Design review of the part shown in the three views and the two pictorial views. Dimensions are in mm from the part's minimum x, y and z. A direction names the side the tool comes from. Round coordinates to 2 decimals unless told otherwise and drop trailing zeros. Write each loop counter-clockwise with the first axis right and the second up, starting at its lowest first coordinate (ties: lowest second). Pieces come first, ordered by that corner, then holes. Notation, with made-up numbers: (-40, -33.75) - (-16, -33.75) arc R22 ccw to (-16, -11.75) - close; hole circle Ø5 at (50.5, 78.5). An arc over 180 degrees is marked (long way). Use one line per item in the form item = value.
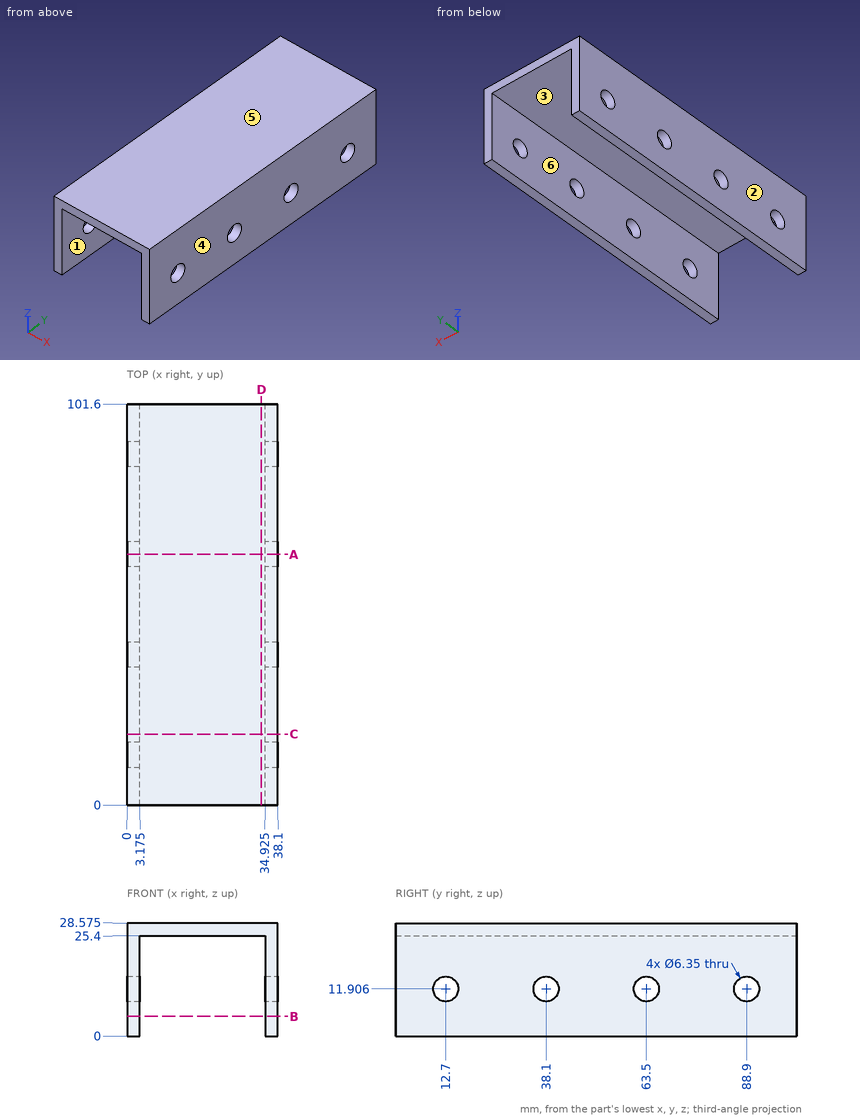
Q1. Draft analysis for pull direction X (two halves, no side actions). For the marked faces 3, 4, 5 and 6, state which applies: released by +X, released by -X, zero draft, split by the parting line, or undercut.
Calculated:
face_3 = undercut
face_4 = released by +X
face_5 = zero draft
face_6 = undercut
Q2. For P1, Ø4, axis at y = 63.5, z = 11.91, coming from the +X side; P2, Ø9.5, axis at x = 22.5, y = 33, coming from the -Z side, all flat-tipped, find the tip position at first contact; note any pin that passes through.
Calculated:
P1 = through
P2 = 25.4
Q3. We need section A-A on y = 63.5. Write out the cut boundary in (x, z) (1 decimal), then the cut area to 3 significant figures.
Calculated:
outline = (0, 0) - (3.2, 0) - (3.2, 8.7) - (0, 8.7) - close; (0, 15.1) - (3.2, 15.1) - (3.2, 25.4) - (34.9, 25.4) - (34.9, 15.1) - (38.1, 15.1) - (38.1, 28.6) - (0, 28.6) - close; (34.9, 0) - (38.1, 0) - (38.1, 8.7) - (34.9, 8.7) - close
area = 242 mm2
Q4. To check wall thickness, follow line 1 along X through (y, z) = (17.5, 5.5) (1 decimal); line 2 along Z through (x, y) = (16, 67.5) (1 decimal); line 3 along Y through (x, z) = (2, 13.5) (1 decimal). State the ranges of each line that lie inside material, in increasing order. Write a range as from..to.
Calculated:
line_1 = 0..3.2, 34.9..38.1
line_2 = 25.4..28.6
line_3 = 0..10, 15.4..35.4, 40.8..60.8, 66.2..86.2, 91.6..101.6
Q5. We need section C-C on y = 18. Write out the cut boundary in (x, z) (1 decimal).
Calculated:
outline = (0, 0) - (3.2, 0) - (3.2, 25.4) - (34.9, 25.4) - (34.9, 0) - (38.1, 0) - (38.1, 28.6) - (0, 28.6) - close
Q6. Machinability: for the marked faces 1 and 2, which of the approach directions +Z, -Z, +X, -X, +Y, -Y give a long, thin tool a straight path to every point of the face, cutting with its end or side? Answer none if there is none.
Calculated:
face_1 = -Z, +Y, -Y
face_2 = +Z, -Z, -X, +Y, -Y
Q7. We need section B-B on z = 5. Write out the cut boundary in (x, y) (1 decimal), then the cut area to 3 significant figures.
Calculated:
outline = (0, 0) - (3.2, 0) - (3.2, 101.6) - (0, 101.6) - close; (34.9, 0) - (38.1, 0) - (38.1, 101.6) - (34.9, 101.6) - close
area = 645 mm2
Q8. We need section D-D on x = 34. Write out the cut boundary in (y, z) (1 decimal).
Calculated:
outline = (0, 25.4) - (101.6, 25.4) - (101.6, 28.6) - (0, 28.6) - close
